```python
from build123d import *

# Parameters (mm, degrees)
SKETCH1_W           = 50
SKETCH1_H           = 36
SKETCH1_R           = 1.25
SKETCH1_R_2         = 1.7
BOSS_EXTRUDE1_DEPTH = 1
SKETCH2_R           = 4
SKETCH2_R_2         = 1.5
BOSS_EXTRUDE2_DEPTH = 8.525


with BuildPart() as part:
    # Sketch1 → Boss-Extrude1 (new body)
    with BuildSketch(Plane(origin=(0, 0, 0), x_dir=(1, 0, 0), z_dir=(0, 1, 0))):
        with Locations((25, 18)):
            Rectangle(SKETCH1_W, SKETCH1_H)
        with Locations((13, 6.5)):
            Circle(SKETCH1_R, mode=Mode.SUBTRACT)
        with Locations((5, 5)):
            Circle(SKETCH1_R_2, mode=Mode.SUBTRACT)
        with Locations((5, 31)):
            Circle(SKETCH1_R_2, mode=Mode.SUBTRACT)
        with Locations((45, 31)):
            Circle(SKETCH1_R_2, mode=Mode.SUBTRACT)
        with Locations((45, 5)):
            Circle(SKETCH1_R_2, mode=Mode.SUBTRACT)
        with Locations((23, 6.5)):
            Circle(SKETCH1_R, mode=Mode.SUBTRACT)
        with Locations((33, 6.5)):
            Circle(SKETCH1_R, mode=Mode.SUBTRACT)
        with Locations((23, 16.5)):
            Circle(SKETCH1_R, mode=Mode.SUBTRACT)
        with Locations((33, 16.5)):
            Circle(SKETCH1_R, mode=Mode.SUBTRACT)
        with Locations((23, 26.5)):
            Circle(SKETCH1_R, mode=Mode.SUBTRACT)
        with Locations((33, 26.5)):
            Circle(SKETCH1_R, mode=Mode.SUBTRACT)
        with Locations((13, 16.5)):
            Circle(SKETCH1_R, mode=Mode.SUBTRACT)
        with Locations((13, 26.5)):
            Circle(SKETCH1_R, mode=Mode.SUBTRACT)
    extrude(amount=BOSS_EXTRUDE1_DEPTH)

    # Sketch2 → Boss-Extrude2 (add)
    with BuildSketch(Plane(origin=(0, 1, 0), x_dir=(1, 0, 0), z_dir=(0, 1, 0))):
        with Locations((13, 26.5)):
            Circle(SKETCH2_R)
        with Locations((13, 26.5)):
            Circle(SKETCH2_R_2, mode=Mode.SUBTRACT)
        with Locations((23, 26.5)):
            Circle(SKETCH2_R)
        with Locations((23, 26.5)):
            Circle(SKETCH2_R_2, mode=Mode.SUBTRACT)
        with Locations((33, 26.5)):
            Circle(SKETCH2_R)
        with Locations((33, 26.5)):
            Circle(SKETCH2_R_2, mode=Mode.SUBTRACT)
        with Locations((23, 16.5)):
            Circle(SKETCH2_R)
        with Locations((23, 16.5)):
            Circle(SKETCH2_R_2, mode=Mode.SUBTRACT)
        with Locations((33, 16.5)):
            Circle(SKETCH2_R)
        with Locations((33, 16.5)):
            Circle(SKETCH2_R_2, mode=Mode.SUBTRACT)
        with Locations((23, 6.5)):
            Circle(SKETCH2_R)
        with Locations((23, 6.5)):
            Circle(SKETCH2_R_2, mode=Mode.SUBTRACT)
        with Locations((33, 6.5)):
            Circle(SKETCH2_R)
        with Locations((33, 6.5)):
            Circle(SKETCH2_R_2, mode=Mode.SUBTRACT)
        with Locations((13, 16.5)):
            Circle(SKETCH2_R)
        with Locations((13, 16.5)):
            Circle(SKETCH2_R_2, mode=Mode.SUBTRACT)
        with Locations((13, 6.5)):
            Circle(SKETCH2_R)
        with Locations((13, 6.5)):
            Circle(SKETCH2_R_2, mode=Mode.SUBTRACT)
    extrude(amount=BOSS_EXTRUDE2_DEPTH)


solid = part.part
```
Here's how the part is built. I have some questions about the finished solid (model axes, mm). A direction names the side the tool comes from. Coordinates: 2 decimals unless noted, no trailing zeros. Order: outer loops, then holes, each group sorted by start corner. A loop starts at its lowest first (then second) coordinate and runs counter-clockwise, first axis right, second up.
Item 1: Which directions (+Z, -Z, +X, -X, +Y, -Y) give clear straight access to the entire face, cutting with the end or side of a thin tool? Please do faces 3 (the face through (25, 9.525, -7)), 4 (the face through (29.8, 5.2, -4.1)).
Response values:
face 3: +Z, -Z, +X, -X, +Y
face 4: +Y
Item 2: I need wall thicknesses on probe 1 along Z at (x, y) = (45, 0.4); probe 2 along Z at (x, y) = (33, 6); probe 3 along X at (y, z) = (4, -16.5). Which ranges of each line are inside material? Lowest first, please.
Response values:
probe 1: z = -36 to -32.7, -29.3 to -6.7, -3.3 to 0
probe 2: z = -30.5 to -28, -25 to -22.5, -20.5 to -18, -15 to -12.5, -10.5 to -8, -5 to -2.5
probe 3: x = 9 to 11.5, 14.5 to 17, 19 to 21.5, 24.5 to 27, 29 to 31.5, 34.5 to 37
Item 3: If we section it at B-B, the plane z = -14: List the corners of the cut face in (x, y) for me (1 decimal).
Response values:
outline: (0, 0) - (50, 0) - (50, 1) - (36.1, 1) - (36.1, 9.5) - (29.9, 9.5) - (29.9, 1) - (26.1, 1) - (26.1, 9.5) - (19.9, 9.5) - (19.9, 1) - (16.1, 1) - (16.1, 9.5) - (9.9, 9.5) - (9.9, 1) - (0, 1) - close
Item 4: If we section it at C-C, the plane x = 26: List the corners of the cut face in (y, z) for me (3 decimals), then the cut area to 3 significant figures.
Response values:
outline: (0, -36) - (1, -36) - (1, -29.146) - (9.525, -29.146) - (9.525, -23.854) - (1, -23.854) - (1, -19.146) - (9.525, -19.146) - (9.525, -13.854) - (1, -13.854) - (1, -9.146) - (9.525, -9.146) - (9.525, -3.854) - (1, -3.854) - (1, 0) - (0, 0) - close
area: 171 mm2
Item 5: If we section it at A-A, the plane y = 2.25: Give the number of separate pieces and of enclosed holes in the cut face, then the cut area to 3 significant figures.
Response values:
separate pieces: 9
enclosed holes: 9
area: 389 mm2
Item 6: I'm going to push flat-ended pins straight in: pin 1 Ø2 at (x, z) = (13, -6.5) entering from -Y; pin 2 Ø1.5 at (x, z) = (19.5, -23) entering from +Y; pin 3 Ø4 at (x, z) = (33, -6.5) entering from -Y. Where does each tip first touch, or does it pass through?
Response values:
pin 1: passes through
pin 2: stops at y = 1
pin 3: stops at y = 0
Item 7: Thinking about a two-plate mould opening in Z: for faces 1 (the face through (50, 0.5, -17.7)), 2 (the face through (12.479, 5.203, -30.466)), which applies, pulls with the +Z half, pulls with the -Z half, needs draft (parallel to the pull), parting line crosses it, or undercut?
Response values:
face 1: needs draft
face 2: undercut
